from build123d import *

# Parameters (mm, degrees)
F0_W     = 838.2
F0_H     = 2438.4
F1_DEPTH = 50.8
F2_W     = 63.5
F2_H     = 2438.4
F3_DEPTH = 203.2
F4_W     = 152.4
F4_H     = 254
F5_DEPTH = 38.1
F6_W     = 304.8
F6_H     = 254
F7_DEPTH = 38.1


with BuildPart() as f1:
    # F0 (on Right) → F1 (new body)
    with BuildSketch(Plane.YZ):
        Rectangle(F0_W, F0_H)
    extrude(amount=F1_DEPTH)

    # F2 (on face) → F3 (join)
    with BuildSketch(Plane(origin=(0, 0, 0), x_dir=(0, -1, 0), z_dir=(-1, 0, 0))):
        with Locations((387.35, 0)):
            Rectangle(F2_W, F2_H)
    extrude(amount=F3_DEPTH)

    # F4 (on face) → F5 (join)
    with BuildSketch(Plane.XZ.offset(419.1)):
        with Locations((-25.4, 939.8)):
            Rectangle(F4_W, F4_H)
    extrude(amount=F5_DEPTH)

    # F6 (on face) → F7 (join)
    with BuildSketch(Plane.YZ.offset(50.8)):
        with Locations((-304.8, 939.8)):
            Rectangle(F6_W, F6_H)
    extrude(amount=F7_DEPTH)


solid = f1.part
Design review of the part built by this model. Coordinates are the model's own, in mm. A direction names the side the tool comes from. Round coordinates to 2 decimals unless told otherwise and drop trailing zeros. Write each loop counter-clockwise with the first axis right and the second up, starting at its lowest first coordinate (ties: lowest second). Pieces come first, ordered by that corner, then holes. Notation, with made-up numbers: (3.25, 60) -> (19.25, 60) arc R20 ccw to (19.25, 80) -> close; hole circle Ø11 at (-16, -39.75). An arc over 180 degrees is marked (long way). One line per item, written item: value. Start each with the question number.
Q1. Tool access review of faces 1 (the face through (88.9, -307, 942)), 2 (the face through (0, 26, 17)): name each direction out of +Z, -Z, +X, -X, +Y, -Y from which nothing blocks a thin tool from reaching the whole face with its end or side.
Q2. To check wall thickness, follow probe 1 along Y at (x, z) = (-185, 686); probe 2 along X at (y, z) = (112, 638); probe 3 along X at (y, z) = (-210, 824.5). State the ranges of each line that lie inside material, in increasing order.
Q3. Add section A-A (y = -189). Give the boundary of the cut face in (x, z).
Q4. Insertion check: P1, Ø4, axis at x = -43.5, z = 902.5, coming from the +Y side; P2, Ø5, axis at y = -309.5, z = 356, coming from the +X side; P3, Ø11.5, axis at y = -429.5, z = 970, coming from the -X side. Each pin has a flat end and moves straight along its axis. Give the tip position at first contact, or say it passes through.
Q5. Add section D-D (z = 93.5). Give the boundary of the cut face in (x, y).
Q6. Add section C-C (z = 918.5). Give the boundary of the cut face in (x, y), then the cut area to 3 significant figures.
Q7. Add section B-B (x = -71.5). Give the boundary of the cut face in (y, z).
Response:
1. face 1: +Z, -Z, +X, +Y, -Y
1. face 2: +Z, -Z, -X, +Y
2. probe 1: y = -419.1 to -355.6
2. probe 2: x = 0 to 50.8
2. probe 3: x = 0 to 88.9
3. outline: (0, -1219.2) -> (50.8, -1219.2) -> (50.8, 812.8) -> (88.9, 812.8) -> (88.9, 1066.8) -> (50.8, 1066.8) -> (50.8, 1219.2) -> (0, 1219.2) -> close
4. P1: stops at y = -355.6
4. P2: stops at x = 50.8
4. P3: stops at x = -101.6
5. outline: (-203.2, -419.1) -> (50.8, -419.1) -> (50.8, 419.1) -> (0, 419.1) -> (0, -355.6) -> (-203.2, -355.6) -> close
6. outline: (-203.2, -419.1) -> (-101.6, -419.1) -> (-101.6, -457.2) -> (88.9, -457.2) -> (88.9, -152.4) -> (50.8, -152.4) -> (50.8, 419.1) -> (0, 419.1) -> (0, -355.6) -> (-203.2, -355.6) -> close
6. area: 72,900 mm^2
7. outline: (-457.2, 812.8) -> (-419.1, 812.8) -> (-419.1, -1219.2) -> (-355.6, -1219.2) -> (-355.6, 1219.2) -> (-419.1, 1219.2) -> (-419.1, 1066.8) -> (-457.2, 1066.8) -> close
